For this review, take the finished solid that the model builds, in its own axes (mm). Face numbers are marked on the shaded views. Give positions to 0.01 mm unless a question says otherwise; leave off trailing zeros. Loops run counter-clockwise (first coordinate to the right, second up) from the corner with the lowest first, then second, coordinate; pieces in that order, holes last. Notation, with made-up numbers: (76, 75) - (111, 75) arc R4 cw to (111, 80) - close; hole circle Ø11 at (-6.5, 36.25). An arc over 180 degrees is marked (long way). Answer as CSV lines item,"result".
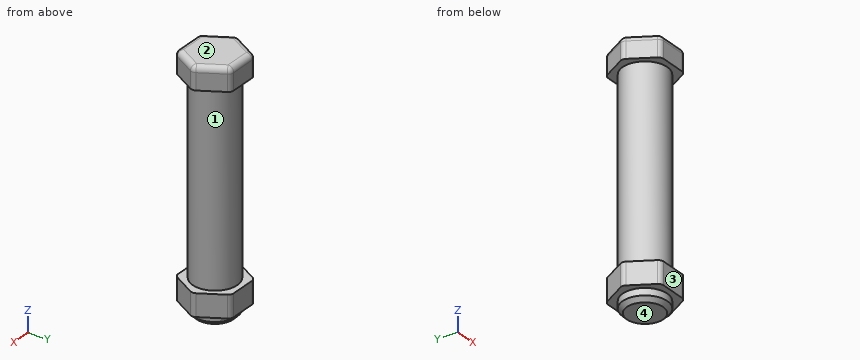
from build123d import *

# Parameters (mm, degrees)
EXTRUDE_1_DEPTH = 4
SKETCH_2_R      = 4
EXTRUDE_2_DEPTH = 34
EXTRUDE_3_DEPTH = 4
SKETCH_4_W      = 4
SKETCH_4_H      = 2
CHAMFER_1_SIZE  = 0.75
FILLET_1_R      = 1


with BuildPart() as part:
    # 草图1 → 凸台-拉伸1 (new body)
    with BuildSketch(Plane.XY.offset(21)):
        Polygon((-2.886751346, -5), (2.886751346, -5), (5.773502692, 0), (2.886751346, 5), (-2.886751346, 5), (-5.773502692, 0), align=None)
    extrude(amount=-EXTRUDE_1_DEPTH)

    # 草图2 → 凸台-拉伸2 (add)
    with BuildSketch(Plane(origin=(0, 0, 17), x_dir=(-1, 0, 0), z_dir=(0, 0, -1))):
        Circle(SKETCH_2_R)
    extrude(amount=EXTRUDE_2_DEPTH)

    # 草图3 → 凸台-拉伸3 (add)
    with BuildSketch(Plane.XY.offset(-17)):
        Polygon((-2.886751346, -5), (2.886751346, -5), (5.773502692, 0), (2.886751346, 5), (-2.886751346, 5), (-5.773502692, 0), align=None)
    extrude(amount=-EXTRUDE_3_DEPTH)

    # 草图4 → 旋转1 (revolve)
    with BuildSketch(Plane.XZ, mode=Mode.PRIVATE) as revolve_1_sk:
        with Locations((2, -22)):
            Rectangle(SKETCH_4_W, SKETCH_4_H)
    revolve(revolve_1_sk.sketch.rotate(Axis((0, 0, -21), (0, 0, -1)), 180), axis=Axis((0, 0, -21), (0, 0, -1)))

    # 倒角1
    chamfer_1_edges = [part.edges().sort_by_distance(p)[0] for p in [
        (4, 0, -23),
    ]]
    chamfer(chamfer_1_edges, length=CHAMFER_1_SIZE)

    # 圆角1
    fillet_1_edges = [part.edges().sort_by_distance(p)[0] for p in [
        (-5.773502692, 0, 19),
        (-2.886751346, 5, 19),
        (2.886751346, 5, 19),
        (5.773502692, 0, 19),
        (2.886751346, -5, 19),
        (-2.886751346, -5, 19),
        (-2.886751346, -5, -19),
        (-5.773502692, 0, -19),
        (-2.886751346, 5, -19),
        (2.886751346, 5, -19),
        (5.773502692, 0, -19),
        (2.886751346, -5, -19),
        (-4.330127019, 2.5, 21),
        (0, 5, 21),
        (4.330127019, 2.5, 21),
        (4.330127019, -2.5, 21),
        (0, -5, 21),
        (-4.330127019, -2.5, 21),
    ]]
    fillet(fillet_1_edges, radius=FILLET_1_R)


solid = part.part
1) Insertion check: P1, Ø2, axis at y = 0, z = 7, coming from the -X side; P2, Ø5, axis at x = 3.5, z = -13, coming from the -Y side; P3, Ø6, axis at x = -1.5, z = 10, coming from the +Y side. Each pin has a flat end and moves straight along its axis. Give the tip position at first contact, or say it passes through.
From the geometry:
P1,"stops at x = -4"
P2,"stops at y = -3.87"
P3,"stops at y = 4"
2) Wall thickness on line 1 (Z direction, x = -3.5, y = 2); line 2 (Y direction, x = 0, z = 15.5); line 3 (Z direction, x = 4.75, y = 1.5): over which ranges is each line inside the solid? List them lowest first. Write a range as from..to.
From the geometry:
line 1,"z = -21..-17, 17..21"
line 2,"y = -4..4"
line 3,"z = -21..-17, 17..20.5"
3) Consider section B-B on z = -3.5. Write out the cut boundary in (x, y), and give its area (3 significant figures).
From the geometry:
outline,"circle Ø8 at (0, 0)"
area,"50.3 mm^2"
4) Consider section A-A on x = 0. Write out the cut boundary in (y, z).
From the geometry:
outline,"(-5, -21) - (-4, -21) - (-4, -22.25) - (-3.25, -23) - (3.25, -23) - (4, -22.25) - (4, -21) - (5, -21) - (5, -17) - (4, -17) - (4, 17) - (5, 17) - (5, 20) arc R1 ccw to (4, 21) - (-4, 21) arc R1 ccw to (-5, 20) - (-5, 17) - (-4, 17) - (-4, -17) - (-5, -17) - close"
5) Draft analysis for pull direction Z (two halves, no side actions). For the marked faces 1, 2, 3 and 4, state which applies: pulls with the +Z half, pulls with the -Z half, needs draft (parallel to the pull), parting line crosses it, or undercut.
From the geometry:
face 1,"undercut"
face 2,"pulls with the +Z half"
face 3,"needs draft"
face 4,"pulls with the -Z half"
